Can you work these out from the model? Positions are in its coordinate system, mm. A direction names the side the tool comes from. Coordinates: 2 decimals unless noted, no trailing zeros. Write each loop counter-clockwise with the first axis right and the second up, starting at its lowest first coordinate (ties: lowest second). Pieces come first, ordered by that corner, then holes.
Autodesk Fusion 360 part; units mm, degrees
sketch "Sketch1" plane through (0, 0, 0) normal (0, 0, 1) x (1, 0, 0)
  circle A0 centre (0, 0) radius 33.5
  dimension "d1" = 67
extrude "Extrude1" add sketch "Sketch1" against normal blind 25
sketch "Sketch2" plane through (0, 0, 0) normal (0, 0, 1) x (1, 0, 0)
  circle A0 centre (0, 0) radius 4.7
  circle A1 centre (0, 0) radius 2.75
  line L0 (2.75, 1.875) -> (-2.75, 1.875)
  line L1 (-2.75, 1.875) -> (-2.75, -1.875)
  line L2 (-2.75, -1.875) -> (2.75, -1.875)
  line L3 (2.75, -1.875) -> (2.75, 1.875)
  line L4 (2.75, 1.875) -> (-2.75, -1.875) construction
  line L5 (-2.75, 1.875) -> (2.75, -1.875) construction
  dimension "d4" = 9.4
  dimension "d7" = 5.5
  dimension "d8" = 3.75
extrude "Extrude2" add sketch "Sketch2" along normal blind 4 contours A0 | A1 L0 L2 | A1 L2 L3 | A1 L0 L3 | A1 L0 | A1 L2 | A1 L0 L1 | A1 L1 L2
extrude "Extrude3" cut sketch "Sketch2" along normal blind 7 and the other way blind 20 contours A1 L0 L2
sketch "Sketch3" plane through (0, 0, 0) normal (0, 0, 1) x (1, 0, 0)
  circle A0 centre (0, 0) radius 4.7
  circle A1 centre (0, 0) radius 33.5
  circle A2 centre (0, 0) radius 22.5
  line L0 (-2.0117, 1.875) -> (2.0117, 1.875)
  arc A3 (2.0117, -1.875) -> (2.0117, 1.875) centre (0, 0) ccw
  line L1 (2.0117, -1.875) -> (-2.0117, -1.875)
  arc A4 (-2.0117, 1.875) -> (-2.0117, -1.875) centre (0, 0) ccw
  circle A5 centre (0, 0) radius 4.7
  dimension "d13" = 45
extrude "Extrude4" cut sketch "Sketch3" against normal blind 11 contours A2
1. If we section it at D-D, the plane z = -18.75: List the corners of the cut face in (x, y) for me (3 decimals), plus the area to 3 significant figures.
2. I'm going to push flat-ended pins straight in: P1, Ø12, axis at x = 7.5, y = 22, coming from the +Z side; P2, Ø2, axis at x = -2.5, z = -10, coming from the +Y side; P3, Ø3, axis at x = 13.5, z = -2.5, coming from the +Y side. Where does each tip first touch, or does it pass through?
3. If we section it at C-C, the plane y = 0: List the corners of the cut face in (x, z) for me.
4. Which directions (+Z, -Z, +X, -X, +Y, -Y) give clear straight access to the entire face, cutting with the end or side of a thin tool? Please do faces 4 (the face through (-0.1, 2.2, 4)), 5 (the face through (-2.75, -0.03, -8.17)).
5. We'd pull the mould along Y, two halves only. Please class faces 1 (the face through (-1.02, -4.59, -3.39)), 2 (the face through (0, 0, -25)), 3 (the face through (-7.262, -32.703, -12.325)): released by +Y, released by -Y, zero draft, split by the parting line, or undercut.
6. If we section it at A-A, the plane z = -7.75: List the corners of the cut face in (x, y) for me (3 decimals).
7. If we section it at B-B, the plane x = 0: List the corners of the cut face in (y, z) for me (3 decimals).
8. If I drill on L1, parallel to Y at x = 0, z = -5.25 (3 decimals); L2, parallel to Z at x = 17.5, y = -11.5; L3, parallel to Z at x = 20.5, y = -10, over which ranges is the centre line in solid material (lowest first)?
Answers:
1. outline: circle Ø67 at (0, 0); hole (-2.012, -1.875) - (2.012, -1.875) arc R2.75 ccw to (2.012, 1.875) - (-2.012, 1.875) arc R2.75 ccw to start
1. area: 3,510 mm2
2. P1: stops at z = 0
2. P2: stops at y = 33.47
2. P3: stops at y = 31.28
3. outline: (-33.5, -25) - (33.5, -25) - (33.5, 0) - (22.5, 0) - (22.5, -11) - (4.7, -11) - (4.7, 4) - (2.75, 4) - (2.75, -20) - (-2.75, -20) - (-2.75, 4) - (-4.7, 4) - (-4.7, -11) - (-22.5, -11) - (-22.5, 0) - (-33.5, 0) - close
4. face 4: +Z, +X, -X, +Y, -Y
4. face 5: +Z
5. face 1: undercut
5. face 2: zero draft
5. face 3: split by the parting line
6. outline: circle Ø67 at (0, 0); circle Ø9.4 at (0, 0); hole circle Ø45 at (0, 0); hole (-2.012, -1.875) - (2.012, -1.875) arc R2.75 ccw to (2.012, 1.875) - (-2.012, 1.875) arc R2.75 ccw to start
7. outline: (-33.5, -25) - (33.5, -25) - (33.5, 0) - (22.5, 0) - (22.5, -11) - (4.7, -11) - (4.7, 4) - (1.875, 4) - (1.875, -20) - (-1.875, -20) - (-1.875, 4) - (-4.7, 4) - (-4.7, -11) - (-22.5, -11) - (-22.5, 0) - (-33.5, 0) - close
8. L1: y = -33.5 to -22.5, -4.7 to -1.875, 1.875 to 4.7, 22.5 to 33.5
8. L2: z = -25 to -11
8. L3: z = -25 to 0
